Model file for the job. Use its own axes, mm. A direction names the side the tool comes from. Give positions to 0.01 mm unless a question says otherwise; leave off trailing zeros. Loops run counter-clockwise (first coordinate to the right, second up) from the corner with the lowest first, then second, coordinate; pieces in that order, holes last. Notation, with made-up numbers: M 26.5,21.25 L 56.5,21.25 A29 ccw 56.5,45.25 Z; hole C 50,23 d5. An arc over 180 degrees is marked long. Answer in a Markdown table with one row per item.
```python
from build123d import *

# Parameters (mm, degrees)
SKETCH1_R               = 2.25
BOSS_EXTRUDE1_DEPTH     = 5
SKETCH2_W               = 52.5
SKETCH2_H               = 52.5
SKETCH2_W_2             = 42.5
SKETCH2_H_2             = 42.5
BOSS_EXTRUDE2_DEPTH     = 40
BOSS_EXTRUDE3_DEPTH     = 36
CUT_EXTRUDE2_DEPTH      = 121.157448791
CUT_EXTRUDE2_DEPTH_BACK = 121.157448791
SKETCH6_R               = 2.5
CUT_EXTRUDE3_DEPTH      = 127.97834461
CUT_EXTRUDE3_DEPTH_BACK = 127.97834461
SKETCH7_R               = 2.5
SKETCH8_W               = 40
SKETCH8_H               = 36.5
CUT_EXTRUDE4_DEPTH      = 24


with BuildPart() as part:
    # Sketch1 → Boss-Extrude1 (new body)
    with BuildSketch(Plane.XY):
        Polygon((0, 30), (-9.25, 30), (-9.25, 82.5), (43.25, 82.5), (43.25, 30), (34, 30), (34, 0), (0, 0), align=None)
        with Locations((4.75, 25.25)):
            Circle(SKETCH1_R, mode=Mode.SUBTRACT)
        with Locations((29.25, 25.25)):
            Circle(SKETCH1_R, mode=Mode.SUBTRACT)
        with Locations((29.25, 4.75)):
            Circle(SKETCH1_R, mode=Mode.SUBTRACT)
        with Locations((4.75, 4.75)):
            Circle(SKETCH1_R, mode=Mode.SUBTRACT)
    extrude(amount=BOSS_EXTRUDE1_DEPTH)

    # Sketch2 → Boss-Extrude2 (add)
    with BuildSketch(Plane.XY.offset(5)):
        with Locations((17, 56.25)):
            Rectangle(SKETCH2_W, SKETCH2_H)
        with Locations((17, 56.25)):
            Rectangle(SKETCH2_W_2, SKETCH2_H_2, mode=Mode.SUBTRACT)
    extrude(amount=BOSS_EXTRUDE2_DEPTH)

    # Sketch5 → Boss-Extrude3 (add)
    with BuildSketch(Plane.XY.offset(45)):
        Polygon((43.25, 82.5), (43.25, 30), (13.25, 30), (13.25, 35), (38.25, 35), (38.25, 77.5), (13.25, 77.5), (13.25, 82.5), align=None)
    extrude(amount=BOSS_EXTRUDE3_DEPTH)

    # Sketch6 → Cut-Extrude2 (cut, two sides: drawn at the far end of the back side and taken through both)
    with BuildSketch(Plane.XZ.offset(-77.5).offset(-CUT_EXTRUDE2_DEPTH_BACK)):
        with Locations(Location((20.75, 73.5, 0), (0, 0, 270))):
            Circle(SKETCH6_R)
    extrude(amount=CUT_EXTRUDE2_DEPTH + CUT_EXTRUDE2_DEPTH_BACK, mode=Mode.SUBTRACT)

    # Sketch7 → Cut-Extrude3 (cut, two sides: drawn at the far end of the back side and taken through both)
    with BuildSketch(Plane(origin=(43.25, 0, 0), x_dir=(0, 0, -1), z_dir=(1, 0, 0)).offset(-CUT_EXTRUDE3_DEPTH_BACK)):
        with Locations(Location((-71, 56.25, 0), (0, 0, 90))):
            Circle(SKETCH7_R)
    extrude(amount=CUT_EXTRUDE3_DEPTH + CUT_EXTRUDE3_DEPTH_BACK, mode=Mode.SUBTRACT)

    # Sketch8 → Cut-Extrude4 (cut)
    with BuildSketch(Plane.ZY.offset(9.25)):
        with Locations((25, 56.25)):
            Rectangle(SKETCH8_W, SKETCH8_H)
    extrude(amount=-CUT_EXTRUDE4_DEPTH, mode=Mode.SUBTRACT)


solid = part.part
```
(1) Flat gauge pins, fed straight in: P1, Ø5, axis at y = 43, z = 67.5, coming from the -X side; P2, Ø10, axis at x = -4, y = 74, coming from the +Z side; P3, Ø5, axis at x = 12.5, y = 69.5, coming from the +Z side. Where does each tip first touch, or does it go through?
Established:
| item | result |
|---|---|
| P1 | stops at x = 38.25 |
| P2 | stops at z = 45 |
| P3 | stops at z = 5 |
(2) Saw through at C-C, the plane y = 33. Give the cut face in (x, z), and give its area (3 significant figures).
Established:
| item | result |
|---|---|
| outline | M -9.25,0 L 43.25,0 L 43.25,81 L 13.25,81 L 13.25,45 L -9.25,45 Z; hole C 20.75,73.5 d5 |
| area | 3,420 mm2 |
(3) Mould opens along Y. For faces 1 (the flat face through (17, 0, 2)), 2 (the flat face through (43.25, 57, 40)), 3 (the flat face through (38.25, 56, 42)) say: pulls with the +Y half, pulls with the -Y half, needs draft (parallel to the pull), parting line crosses it, or undercut.
Established:
| item | result |
|---|---|
| face 1 | pulls with the -Y half |
| face 2 | needs draft |
| face 3 | undercut |
(4) Wall check: L1, parallel to Y at x = 41.35, z = 71; L2, parallel to Y at x = -3, z = 29.5; L3, parallel to X at y = 33.5, z = 73.5. Give the ranges that are in metal, low to high.
Established:
| item | result |
|---|---|
| L1 | y = 30 to 53.75, 58.75 to 82.5 |
| L2 | y = 30 to 35, 77.5 to 82.5 |
| L3 | x = 13.25 to 18.25, 23.25 to 43.25 |
(5) Saw through at A-A, the plane x = 4.75. Give the cut face in (y, z).
Established:
| item | result |
|---|---|
| outline | M 0,0 L 2.5,0 L 2.5,5 L 0,5 Z; M 7,0 L 23,0 L 23,5 L 7,5 Z; M 27.5,0 L 82.5,0 L 82.5,45 L 77.5,45 L 77.5,5 L 35,5 L 35,45 L 30,45 L 30,5 L 27.5,5 Z |
(6) Saw through at D-D, the plane z = 22.5. Give the cut face in (x, y).
Established:
| item | result |
|---|---|
| outline | M -9.25,30 L 43.25,30 L 43.25,82.5 L -9.25,82.5 L -9.25,74.5 L -4.25,74.5 L -4.25,77.5 L 38.25,77.5 L 38.25,35 L -4.25,35 L -4.25,38 L -9.25,38 Z |
(7) Saw through at B-B, the plane y = 4.75. Give the cut face in (x, z), and give its area (3 significant figures).
Established:
| item | result |
|---|---|
| outline | M 0,0 L 2.5,0 L 2.5,5 L 0,5 Z; M 7,0 L 27,0 L 27,5 L 7,5 Z; M 31.5,0 L 34,0 L 34,5 L 31.5,5 Z |
| area | 125 mm2 |
(8) Which spindle directions (+Z, -Z, +X, -X, +Y, -Y) get a long thin tool onto all of the face, cutting with end or side? Do faces 4 (the flat face through (-4.25, 76, 25)), 5 (the flat face through (13.25, 32, 63)), 6 (the flat face through (17, 15, 5)), 7 (the flat face through (34, 15, 2)), 8 (the flat face through (-7, 74.5, 25)). Say none if no direction does.
Established:
| item | result |
|---|---|
| face 4 | +Z |
| face 5 | +Z, -X, +Y, -Y |
| face 6 | +Z, +X, -X, -Y |
| face 7 | +Z, -Z, +X, -Y |
| face 8 | +Z, -X |
